Geometry: final body of the model. Coordinates: model frame, mm. A direction names the side the tool comes from. Round coordinates to 2 decimals unless told otherwise and drop trailing zeros. Order: outer loops, then holes, each group sorted by start corner. A loop starts at its lowest first (then second) coordinate and runs counter-clockwise, first axis right, second up. Notation, with made-up numbers: (-28, -25) - (-10, -25) arc R20 cw to (-10, -3) - close; hole circle Ø5 at (-14, 16.5). An arc over 180 degrees is marked (long way). Put each result on its own line as item: value. Start each with the question number.
(1) Pull-direction query (Z, two-part tool) for faces 1 (the face through (0.078, 1.453, 10.075)), 2 (the face through (-0.1, -3.048, 4.3)), 3 (the face through (0, 0, 26.162)); classes: released by +Z, released by -Z, zero draft, split by the parting line, or undercut.
(2) Material intervals for L1, parallel to Y at x = 2, z = 9.75; L2, parallel to Y at x = -2, z = 24.5; L3, parallel to Y at x = -2.75, z = 5.75, sorted ascending. Write a range as [from, to].
(3) Section D-D (y = 4). Output: boundary loops of the cut face in (x, z).
(4) Section A-A (z = 5.25). Output: boundary loops of the cut face in (x, y), and give its area (3 significant figures).
(5) Section B-B (x = 0.75). Count the separate pieces of the cut face and the enclosed holes in it, and give its area (3 significant figures).
(6) Section C-C (y = -1.25). Output: boundary loops of the cut face in (x, z).
(7) Access query for faces 4 (the face through (5.588, 0, 17)), 5 (the face through (3.048, 1, 4)), 6 (the face through (-5.842, 0, 4)), 7 (the face through (-5.588, 0, 17)). Directions: +Z, -Z, +X, -X, +Y, -Y. A direction counts if a zero-diameter tool reaches every point of the face in a straight line with its end or side. Return the directions, or none.
(8) Pin query (flat end, axial travel): P1, Ø0.6, axis at y = 1.778, z = 14.732, coming from the -X side; P2, Ø1.7, axis at y = 1.778, z = 9.652, coming from the +X side. Return the tip coordinate at first contact, or that it passes through.
from build123d import *

# Parameters (mm, degrees)
SKETCH1_W               = 11.684
SKETCH1_H               = 9.652
BOSS_EXTRUDE1_DEPTH     = 7.112
CUT_EXTRUDE1_DEPTH      = 14.336814162
CUT_EXTRUDE1_DEPTH_BACK = 14.336814162
SKETCH2_R               = 1.2065
SKETCH7_W               = 11.176
SKETCH7_H               = 9.144
BOSS_EXTRUDE3_DEPTH     = 19.05
SKETCH9_R               = 0.5334
CUT_EXTRUDE2_DEPTH      = 29.954885943


with BuildPart() as part:
    # Sketch1 → Boss-Extrude1 (new body)
    with BuildSketch(Plane.XY):
        Rectangle(SKETCH1_W, SKETCH1_H)
        Polygon((-4.064, -3.048), (4.064, -3.048), (4.064, -0.381), (3.048, -0.381), (3.048, 3.048), (-3.048, 3.048), (-3.048, -0.381), (-4.064, -0.381), align=None, mode=Mode.SUBTRACT)
    extrude(amount=BOSS_EXTRUDE1_DEPTH)

    # Sketch2 → Cut-Extrude1 (cut, two sides: drawn at the far end of the back side and taken through both)
    with BuildSketch(Plane(origin=(0, 4.826, 0), x_dir=(1, 0, 0), z_dir=(0, 1, 0)).offset(-CUT_EXTRUDE1_DEPTH_BACK)):
        with Locations(Location((0, -2.794, 0), (0, 0, 90))):
            Circle(SKETCH2_R)
    extrude(amount=CUT_EXTRUDE1_DEPTH + CUT_EXTRUDE1_DEPTH_BACK, mode=Mode.SUBTRACT)

    # Sketch7 → Boss-Extrude3 (add)
    with BuildSketch(Plane.XY.offset(7.112)):
        Rectangle(SKETCH7_W, SKETCH7_H)
    extrude(amount=BOSS_EXTRUDE3_DEPTH)

    # Sketch9 → Cut-Extrude2 (cut, through all)
    with BuildSketch(Plane(origin=(5.588, 0, 0), x_dir=(0, 0, -1), z_dir=(1, 0, 0))):
        with Locations((-9.652, -2.54)):
            Circle(SKETCH9_R)
        with Locations((-12.192, -2.54)):
            Circle(SKETCH9_R)
        with Locations((-14.732, -2.54)):
            Circle(SKETCH9_R)
        with Locations((-17.272, -2.54)):
            Circle(SKETCH9_R)
        with Locations((-19.812, -2.54)):
            Circle(SKETCH9_R)
        with Locations((-22.352, -2.54)):
            Circle(SKETCH9_R)
        with Locations((-24.892, -2.54)):
            Circle(SKETCH9_R)
        with Locations((-12.192, 1.778)):
            Circle(SKETCH9_R)
        with Locations((-14.732, 1.778)):
            Circle(SKETCH9_R)
        with Locations((-17.272, 1.778)):
            Circle(SKETCH9_R)
        with Locations((-19.812, 1.778)):
            Circle(SKETCH9_R)
        with Locations((-22.352, 1.778)):
            Circle(SKETCH9_R)
        with Locations((-24.892, 1.778)):
            Circle(SKETCH9_R)
        with Locations((-9.652, 1.778)):
            Circle(SKETCH9_R)
    extrude(amount=-CUT_EXTRUDE2_DEPTH, mode=Mode.SUBTRACT)


solid = part.part
Checks:
1. face 1: undercut
1. face 2: zero draft
1. face 3: released by +Z
2. L1: y = [-4.57, -3.06], [-2.02, 1.25], [2.3, 4.57]
2. L2: y = [-4.57, -2.9], [-2.18, 1.42], [2.14, 4.57]
2. L3: y = [-4.83, -3.05], [3.05, 4.83]
3. outline: (-5.84, 0) - (5.84, 0) - (5.84, 7.11) - (5.59, 7.11) - (5.59, 26.16) - (-5.59, 26.16) - (-5.59, 7.11) - (-5.84, 7.11) - close; hole circle Ø2.41 at (0, 2.79)
4. outline: (-5.84, -4.83) - (5.84, -4.83) - (5.84, 4.83) - (-5.84, 4.83) - close; hole (-4.06, -3.05) - (4.06, -3.05) - (4.06, -0.38) - (3.05, -0.38) - (3.05, 3.05) - (-3.05, 3.05) - (-3.05, -0.38) - (-4.06, -0.38) - close
4. area: 70.2 mm²
5. separate pieces: 3
5. enclosed holes: 14
5. area: 180 mm²
6. outline: (-5.84, 0) - (-4.06, 0) - (-4.06, 7.11) - (4.06, 7.11) - (4.06, 0) - (5.84, 0) - (5.84, 7.11) - (5.59, 7.11) - (5.59, 26.16) - (-5.59, 26.16) - (-5.59, 7.11) - (-5.84, 7.11) - close
7. face 4: +Z, +X, +Y, -Y
7. face 5: -Z
7. face 6: +Z, -Z, -X, +Y, -Y
7. face 7: +Z, -X, +Y, -Y
8. P1: passes through
8. P2: stops at x = 5.59
